Answer from the drawing. Dimensions are ordinates in mm from the lowest x, y and z of the part. Round coordinates to 2 decimals unless told otherwise and drop trailing zeros. Write each loop counter-clockwise with the first axis right and the second up, starting at its lowest first coordinate (ties: lowest second). Pieces come first, ordered by that corner, then holes. Notation, with made-up numbers: M -32,-37.5 L 6,-37.5 A27 ccw 6,0.5 Z; hole C 47.5,36 d3. An arc over 180 degrees is marked long. Answer as CSV lines item,"result". Start each with the question number.
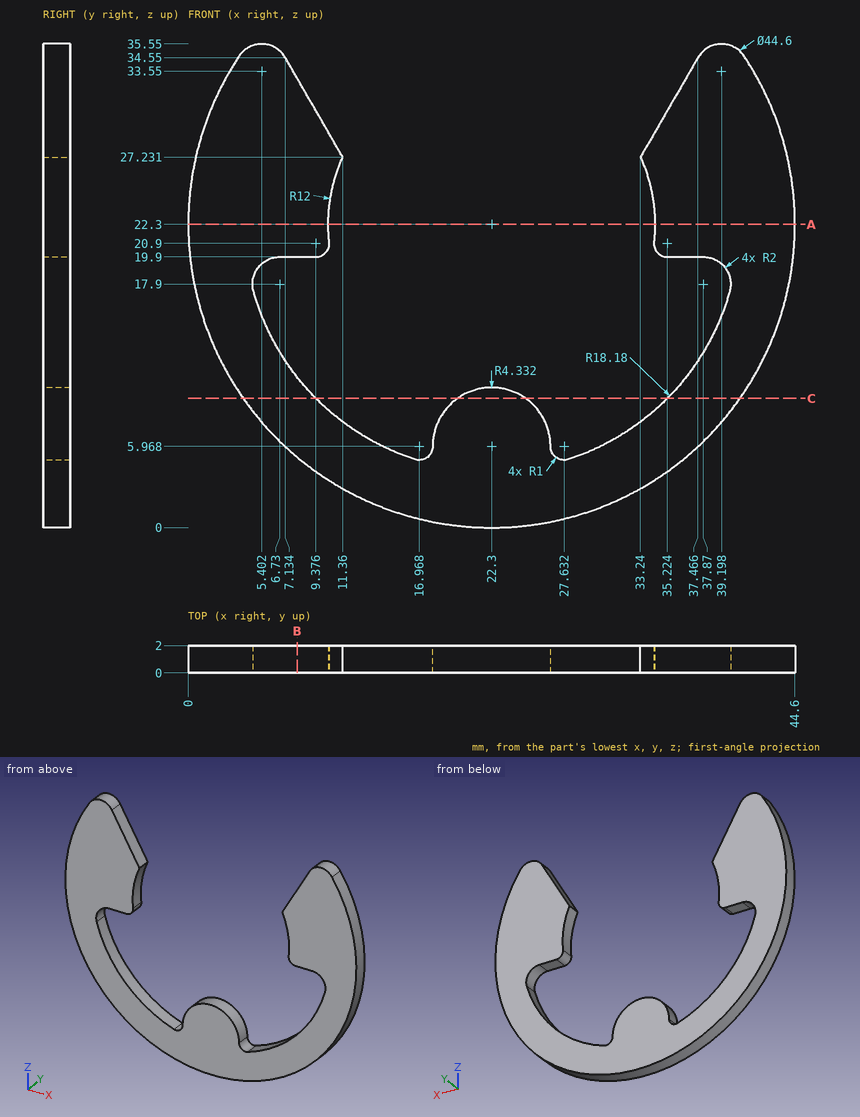
Q1. Straight lines are drawn through the part: L1, parallel to X at y = 1.7, z = 7 (1 decimal); L2, parallel to X at y = 0.5, z = 8.5 (1 decimal); L3, parallel to Z at x = 22.5, y = 0.55 (1 decimal). For each, find the intervals that lie inside material, in ascending order.
Q2. Find section C-C (z = 9.5). Determine the outline of the cut face in (x, y).
Q3. Find section B-B (x = 8). Determine the outline of the cut face in (y, z).
Q4. Find section A-A (z = 22.3). Determine the outline of the cut face in (x, y).
Q5. Each of these flat-tipped pins is pushed along its axis until it touches: P1, Ø1, axis at x = 8.5, y = 1, coming from the -Z side; P2, Ø2, axis at x = 36.5, z = 5.5, coming from the -Y side; P3, Ø1, axis at x = 36.5, y = 1.5, coming from the -Z side (1 decimal); P4, Ø1, axis at y = 0.5, z = 4, coming from the +X side (1 decimal). Where does it stop, or does it pass through?
Reported:
1,L1,"x = 6.1 to 12.5, 18.1 to 26.5, 32.1 to 38.5"
1,L2,"x = 4.8 to 10.5, 18.8 to 25.8, 34.1 to 39.8"
1,L3,"z = 0 to 10.3"
2,outline,"M 4.04,0 L 9.39,0 L 9.39,2 L 4.04,2 Z; M 19.79,0 L 24.81,0 L 24.81,2 L 19.79,2 Z; M 35.21,0 L 40.56,0 L 40.56,2 L 35.21,2 Z"
3,outline,"M 0,5.19 L 2,5.19 L 2,11.07 L 0,11.07 Z; M 0,19.9 L 2,19.9 L 2,33.05 L 0,33.05 Z"
4,outline,"M 0,0 L 10.3,0 L 10.3,2 L 0,2 Z; M 34.3,0 L 44.6,0 L 44.6,2 L 34.3,2 Z"
5,P1,"stops at z = 4.4"
5,P2,"stops at y = 0"
5,P3,"stops at z = 4.7"
5,P4,"stops at x = 35.7"
